Design review of the part built by this model. Coordinates are the model's own, in mm. A direction names the side the tool comes from. Coordinates: 2 decimals unless noted, no trailing zeros. Loops run counter-clockwise (first coordinate to the right, second up) from the corner with the lowest first, then second, coordinate; pieces in that order, holes last. Notation, with made-up numbers: (-9, 33) -> (33, 33) arc R19 cw to (33, 51) -> close; hole circle Ø11 at (75.25, 87). An arc over 180 degrees is marked (long way). Answer as a JSON object with one key per item and string values.
```python
from build123d import *

# Parameters (mm, degrees)
F0_R     = 9
F0_R_2   = 1
F1_DEPTH = 2
F4_DEPTH = 8
F3_R     = 11
F5_DEPTH = 8


with BuildPart() as f1:
    # F0 (on Top) → F1 (new body)
    with BuildSketch(Plane.XY):
        with BuildLine():
            Line((7.3873995355, 21.3588363291), (-3.6126004645, 21.3588363291))
            ThreePointArc((-3.6126004645, 21.3588363291), (-14.2192021823, 16.9654380469), (-18.6126004645, 6.3588363291))
            ThreePointArc((-18.6126004645, 6.3588363291), (-14.2192021823, -4.2477653887), (-3.6126004645, -8.6411636709))
            Line((-3.6126004645, -8.6411636709), (7.3873995355, -8.6411636709))
            ThreePointArc((7.3873995355, -8.6411636709), (10.2158266602, -7.4695907956), (11.3873995355, -4.6411636709))
            Line((11.3873995355, -4.6411636709), (11.3873995355, -2.0833974181))
            ThreePointArc((11.3873995355, -2.0833974181), (12.2455583984, 0.0172016735), (14.3290772311, 0.9160356132))
            Line((14.3290772311, 0.9160356132), (62.8159749994, 1.8588363291))
            Line((62.8159749994, 1.8588363291), (62.8159749994, 10.8588363291))
            Line((62.8159749994, 10.8588363291), (14.3290772311, 11.8016370451))
            ThreePointArc((14.3290772311, 11.8016370451), (12.2455583984, 12.7004709848), (11.3873995355, 14.8010700763))
            Line((11.3873995355, 14.8010700763), (11.3873995355, 17.3588363291))
            ThreePointArc((11.3873995355, 17.3588363291), (10.2158266602, 20.1872634539), (7.3873995355, 21.3588363291))
        make_face()
        with Locations((-3.6126004645, 6.3588363291)):
            Circle(F0_R, mode=Mode.SUBTRACT)
        with Locations((27.1540286045, 6.3588363291)):
            Circle(F0_R_2, mode=Mode.SUBTRACT)
        with Locations((41.830126385, 6.3588363291)):
            Circle(F0_R_2, mode=Mode.SUBTRACT)
        with Locations((54.8330286544, 6.3588363291)):
            Circle(F0_R_2, mode=Mode.SUBTRACT)
    extrude(amount=F1_DEPTH)

    # F4 (add): a face of the model
    f4_faces = [f1.faces().sort_by_distance(p)[0] for p in [
        (16.5282103985, 6.3588363291, 2),
    ]]
    extrude(f4_faces, amount=F4_DEPTH)

    # F3 (on offset) → F5 (cut)
    with BuildSketch(Plane.XY.offset(2)):
        with Locations((-3.6273910664, 6.2710107304)):
            Circle(F3_R)
    extrude(amount=F5_DEPTH, mode=Mode.SUBTRACT)


solid = f1.part
```
1) Add section D-D, the plane x = 27. Give the boundary of the cut face in (y, z), and give its area (3 significant figures).
Completed:
{"outline": "(1.16, 0) -> (5.37, 0) -> (5.37, 10) -> (1.16, 10) -> close; (7.35, 0) -> (11.56, 0) -> (11.56, 10) -> (7.35, 10) -> close", "area": "84.2 mm²"}
2) Add section C-C, the plane z = 3.25. Give the boundary of the cut face in (x, y).
Completed:
{"outline": "(-3.61, -8.64) -> (7.39, -8.64) arc R4 ccw to (11.39, -4.64) -> (11.39, -2.08) arc R3 cw to (14.33, 0.92) -> (62.82, 1.86) -> (62.82, 10.86) -> (14.33, 11.8) arc R3 cw to (11.39, 14.8) -> (11.39, 17.36) arc R4 ccw to (7.39, 21.36) -> (-3.61, 21.36) arc R15 ccw to start; hole circle Ø22 at (-3.63, 6.27); hole circle Ø2 at (27.15, 6.36); hole circle Ø2 at (41.83, 6.36); hole circle Ø2 at (54.83, 6.36)"}
3) Clearance check with flat-ended pins moving along their axes: pin 1 Ø3 at (y, z) = (-3.5, 6) entering from +X; pin 2 Ø1 at (y, z) = (9.5, 7.5) entering from -X; pin 3 Ø1.5 at (y, z) = (18, 5) entering from -X. State where each tip first meets the part, or that it passes through.
Completed:
{"pin 1": "x = 11.39", "pin 2": "x = -18.38", "pin 3": "x = -13.93"}
4) Add section A-A, the plane x = -1. Give the boundary of the cut face in (y, z).
Completed:
{"outline": "(-8.64, 0) -> (-2.25, 0) -> (-2.25, 2) -> (-4.41, 2) -> (-4.41, 10) -> (-8.64, 10) -> close; (14.97, 0) -> (21.36, 0) -> (21.36, 10) -> (16.95, 10) -> (16.95, 2) -> (14.97, 2) -> close"}
5) Add section B-B, the plane y = 9.5. Give the boundary of the cut face in (x, z).
Completed:
{"outline": "(-18.28, 0) -> (-12.05, 0) -> (-12.05, 2) -> (-14.14, 2) -> (-14.14, 10) -> (-18.28, 10) -> close; (4.82, 0) -> (62.82, 0) -> (62.82, 10) -> (6.89, 10) -> (6.89, 2) -> (4.82, 2) -> close"}
6) For faces 4 (the flat face through (11.387, -3, 5)), 5 (the cylindrical face through (-6.012, -4.467, 5.944)), 6 (the flat face through (11.387, 16, 5)), 7 (the flat face through (62.816, 6, 5)), list the 3-axis set-ups (+Z, -Z, +X, -X, +Y, -Y) from which the entire face can be reached by the end or side of a thin tool; tool diameter is ignored.
Completed:
{"face 4": "+Z, -Z, +X, -Y", "face 5": "+Z", "face 6": "+Z, -Z, +X, +Y", "face 7": "+Z, -Z, +X, +Y, -Y"}
7) Wall thickness on probe 1 along Y at (x, z) = (-4, 8); probe 2 along X at (y, z) = (8.5, 2.25); probe 3 along X at (y, z) = (13, 0.5): over which ranges is each line inside the solid? List them lowest first.
Completed:
{"probe 1": "-8.64 to -4.72, 17.26 to 21.35", "probe 2": "-18.46 to -14.4, 7.14 to 62.82", "probe 3": "-17.06 to -9.69, 2.46 to 11.99"}
8) The part is to be moulded in two halves that separate along Y. For faces 1 (the cylindrical face through (10.247, 20.156, 4.93)), 2 (the cylindrical face through (-18.61, 6.69, 4.93)), 3 (the flat face through (-2, -3, 2)), say which applies: pulls with the +Y half, pulls with the -Y half, needs draft (parallel to the pull), parting line crosses it, or undercut.
Completed:
{"face 1": "pulls with the +Y half", "face 2": "parting line crosses it", "face 3": "undercut"}
